Design review of the part built by this model. Coordinates are the model's own, in mm. A direction names the side the tool comes from. Give positions to 0.01 mm unless a question says otherwise; leave off trailing zeros. Write each loop counter-clockwise with the first axis right and the second up, starting at its lowest first coordinate (ties: lowest second). Pieces come first, ordered by that corner, then holes. Notation, with made-up numbers: (28.5, -12.5) - (69.5, -12.5) arc R17 ccw to (69.5, 10.5) - close; hole circle Ø4 at (78, -30). An arc over 180 degrees is marked (long way). Use a Markdown table: item, result. Add a question column.
```python
from build123d import *

# Parameters (mm, degrees)
SKETCH1_W           = 76.2
SKETCH1_H           = 50
BOSS_EXTRUDE1_DEPTH = 3
CUT_EXTRUDE1_DEPTH  = 4


with BuildPart() as part:
    # Sketch1 → Boss-Extrude1 (new body)
    with BuildSketch(Plane(origin=(0, 0, 0), x_dir=(1, 0, 0), z_dir=(0, 1, 0))):
        Rectangle(SKETCH1_W, SKETCH1_H)
    extrude(amount=BOSS_EXTRUDE1_DEPTH)

    # Sketch2 → Cut-Extrude1 (cut, through all)
    with BuildSketch(Plane(origin=(0, 3, 0), x_dir=(1, 0, 0), z_dir=(0, 1, 0))):
        with BuildLine():
            Line((-25.4, 19.8), (25.4, 19.8))
            ThreePointArc((25.4, 19.8), (29.7, 15.5), (25.4, 11.2))
            Line((25.4, 11.2), (-25.4, 11.2))
            ThreePointArc((-25.4, 11.2), (-29.7, 15.5), (-25.4, 19.8))
        make_face()
        with BuildLine():
            Line((-25.4, -19.8), (25.4, -19.8))
            ThreePointArc((25.4, -19.8), (29.7, -15.5), (25.4, -11.2))
            Line((25.4, -11.2), (-25.4, -11.2))
            ThreePointArc((-25.4, -11.2), (-29.7, -15.5), (-25.4, -19.8))
        make_face()
        with BuildLine():
            Line((-12.5, 5.5), (12.5, 5.5))
            ThreePointArc((12.5, 5.5), (18, 0), (12.5, -5.5))
            Line((12.5, -5.5), (-12.5, -5.5))
            ThreePointArc((-12.5, -5.5), (-18, 0), (-12.5, 5.5))
        make_face()
    extrude(amount=-CUT_EXTRUDE1_DEPTH, mode=Mode.SUBTRACT)


solid = part.part
```
(1) Add section B-B (y = 1.25). State the section outline as (x, z) points.
(2) Add section D-D (z = 0). State the section outline as (x, y) points, and give its area (3 significant figures).
(3) Add section C-C (x = 28.5). State the section outline as (y, z) points, and give its area (3 significant figures).
(4) Mouldability with a two-part tool opening along Z and no side actions: class faces 3 (the face through (-1, 1, -25)), 4 (the face through (-38.1, 1, 0)), 5 (the face through (0, 2, 19.8)) as +Z half, -Z half, draft (parallel to the pull), parting line (faces both ways), or undercut.
(5) Tool access review of faces 1 (the face through (-29.7, 1.5, 15.4)), 2 (the face through (-1, 3, -6)): name each direction out of +Z, -Z, +X, -X, +Y, -Y from which nothing blocks a thin tool from reaching the whole face with its end or side.
(6) For line 1 along Z through (x, y) = (-3, 2.4); line 2 along Z through (x, y) = (-16.5, 0.25); line 3 along Z through (x, y) = (-27, 1.85), list the stretches that pass through material, from the lowest coordinate up.
(7) Add section A-A (z = 15.5). State the section outline as (x, y) points, and give its area (3 significant figures).
Answers follow:
| question | item | result |
|---|---|---|
| 1 | outline | (-38.1, -25) - (38.1, -25) - (38.1, 25) - (-38.1, 25) - close; hole (-25.4, -19.8) - (25.4, -19.8) arc R4.3 ccw to (25.4, -11.2) - (-25.4, -11.2) arc R4.3 ccw to start; hole (-25.4, 11.2) - (25.4, 11.2) arc R4.3 ccw to (25.4, 19.8) - (-25.4, 19.8) arc R4.3 ccw to start; hole (-12.5, -5.5) - (12.5, -5.5) arc R5.5 ccw to (12.5, 5.5) - (-12.5, 5.5) arc R5.5 ccw to start |
| 2 | outline | (-38.1, 0) - (-18, 0) - (-18, 3) - (-38.1, 3) - close; (18, 0) - (38.1, 0) - (38.1, 3) - (18, 3) - close |
| 2 | area | 121 mm^2 |
| 3 | outline | (0, -25) - (3, -25) - (3, -18.48) - (0, -18.48) - close; (0, -12.52) - (3, -12.52) - (3, 12.52) - (0, 12.52) - close; (0, 18.48) - (3, 18.48) - (3, 25) - (0, 25) - close |
| 3 | area | 114 mm^2 |
| 4 | face 3 | -Z half |
| 4 | face 4 | draft |
| 4 | face 5 | undercut |
| 5 | face 1 | +Y, -Y |
| 5 | face 2 | +Z, -Z, +X, -X, +Y |
| 6 | line 1 | -25 to -19.8, -11.2 to -5.5, 5.5 to 11.2, 19.8 to 25 |
| 6 | line 2 | -25 to -19.8, -11.2 to -3.77, 3.77 to 11.2, 19.8 to 25 |
| 6 | line 3 | -25 to -19.49, -11.51 to 11.51, 19.49 to 25 |
| 7 | outline | (-38.1, 0) - (-29.7, 0) - (-29.7, 3) - (-38.1, 3) - close; (29.7, 0) - (38.1, 0) - (38.1, 3) - (29.7, 3) - close |
| 7 | area | 50.4 mm^2 |
